Verification items for the finished model (mm, model axes). Face numbers are marked on the shaded views. A direction names the side the tool comes from. Coordinates: 2 decimals unless noted, no trailing zeros. Order: outer loops, then holes, each group sorted by start corner. A loop starts at its lowest first (then second) coordinate and runs counter-clockwise, first axis right, second up. Notation, with made-up numbers: (57.25, 57) -> (79.25, 57) arc R19 cw to (79.25, 87) -> close; hole circle Ø9 at (-7.5, -20). An arc over 180 degrees is marked (long way). Write item = value, one per line. Start each with the question number.
1. Cross-section at B-B on y = -421. Record the cut outline in (x, z), plus the area to 3 significant figures.
2. Thickness scan on line 1 along Z through (x, y) = (487, -606); line 2 along Y through (x, z) = (358, 152.5); line 3 along X through (y, z) = (-537.5, 164). Record the ranges inside material, lowest first. Write a range as from..to.
3. Cross-section at C-C on x = 64. Record the cut outline in (y, z).
4. Cross-section at A-A on z = 359.5. Record the cut outline in (x, y).
5. Go/stop test with a flat-tipped pin: P1, Ø4, axis at x = 268.5, y = -381.5, coming from the -Z side. Record where the tip stops, or that it passes through.
6. Release check for a two-part mould opening along X. For the marked faces 1, 2 and 3 record: +X half, -X half, draft (parallel to the pull), parting line (faces both ways), or undercut.
7. Set-up check for the marked faces 4 and 5: record each of +Z, -Z, +X, -X, +Y, -Y from which the full face is reachable in a straight line by a thin tool's end or side.
from build123d import *

# Parameters (mm, degrees)
SKETCH_2_W           = 559.015307906
SKETCH_2_H           = 680
EXTRUDE_2_DEPTH      = 400
SKETCH_3_OUTSIDE_W   = 754.395
SKETCH_3_OUTSIDE_H   = 875.38
SKETCH_3_OUTSIDE_W_2 = 559.015307906
SKETCH_3_OUTSIDE_H_2 = 490.432891875
CUT_EXTRUDE_1_DEPTH  = 784.744027655
SKETCH_4_W           = 559.015307906
SKETCH_4_H           = 490.432891875
EXTRUDE_3_DEPTH      = 100
SHELL_2_T            = -30
SKETCH_5_W           = 499.015307907
SKETCH_5_H           = 6
CUT_EXTRUDE_2_DEPTH  = 10
SKETCH_6_W           = 499.015307907
SKETCH_6_H           = 6
CUT_EXTRUDE_3_DEPTH  = 10
SKETCH_7_W           = 6
SKETCH_7_H           = 490.432891874
CUT_EXTRUDE_4_DEPTH  = 10


with BuildPart() as part:
    # 草图2 → 凸台-拉伸2 (new body)
    with BuildSketch(Plane(origin=(180.83794206, -79.035754343, 0), x_dir=(1, 0, 0), z_dir=(0, 0, 1))):
        with Locations((101.397699083, -216.026809528)):
            Rectangle(SKETCH_2_W, SKETCH_2_H)
    extrude(amount=EXTRUDE_2_DEPTH)

    # 草图3 outside → 切除-拉伸1 (cut, through all)
    with BuildSketch(Plane(origin=(180.83794206, -79.035754343, 400), x_dir=(1, 0, 0), z_dir=(0, 0, 1))):
        with Locations((101.3975, -216.027)):
            Rectangle(SKETCH_3_OUTSIDE_W, SKETCH_3_OUTSIDE_H)
        with Locations((101.397699083, -310.72828395)):
            Rectangle(SKETCH_3_OUTSIDE_W_2, SKETCH_3_OUTSIDE_H_2, mode=Mode.SUBTRACT)
    extrude(amount=-CUT_EXTRUDE_1_DEPTH, mode=Mode.SUBTRACT)

    # 草图4 → 凸台-拉伸3 (add)
    with BuildSketch(Plane(origin=(180.83794206, -79.035754343, 0), x_dir=(-1, 0, 0), z_dir=(0, 0, -1))):
        with Locations((-101.397699083, -310.72828395)):
            Rectangle(SKETCH_4_W, SKETCH_4_H)
    extrude(amount=EXTRUDE_3_DEPTH)

    # 抽壳2
    shell_2_openings = [part.faces().sort_by_distance(p)[0] for p in [
        (282.235641143, -389.764038294, -100),
    ]]
    offset(amount=SHELL_2_T, openings=shell_2_openings, kind=Kind.INTERSECTION)

    # 草图5 → 切除-拉伸2 (cut)
    with BuildSketch(Plane.XZ.offset(174.547592357)):
        with Locations((282.235641143, -87)):
            Rectangle(SKETCH_5_W, SKETCH_5_H)
    cut_extrude_2 = extrude(amount=-CUT_EXTRUDE_2_DEPTH, mode=Mode.SUBTRACT)

    # 草图6 → 切除-拉伸3 (cut)
    with BuildSketch(Plane.XZ.offset(174.547592357)):
        with Locations((282.235641143, -76)):
            Rectangle(SKETCH_6_W, SKETCH_6_H)
    cut_extrude_3 = extrude(amount=-CUT_EXTRUDE_3_DEPTH, mode=Mode.SUBTRACT)

    # 镜向1: 切除-拉伸2, 切除-拉伸3 across plane
    add(cut_extrude_2.mirror(Plane(origin=(0, -389.764038294, 0), x_dir=(0, 0, 1), z_dir=(0, -1, 0))), mode=Mode.SUBTRACT)
    add(cut_extrude_3.mirror(Plane(origin=(0, -389.764038294, 0), x_dir=(0, 0, 1), z_dir=(0, -1, 0))), mode=Mode.SUBTRACT)

    # 草图7 → 切除-拉伸4 (cut)
    with BuildSketch(Plane.XY.offset(400)):
        with Locations((548.743295096, -389.764038294)):
            Rectangle(SKETCH_7_W, SKETCH_7_H)
    cut_extrude_4 = extrude(amount=-CUT_EXTRUDE_4_DEPTH, mode=Mode.SUBTRACT)

    # 镜向2: 切除-拉伸4 across plane
    add(cut_extrude_4.mirror(Plane.ZY.offset(-282.235641143)), mode=Mode.SUBTRACT)


solid = part.part
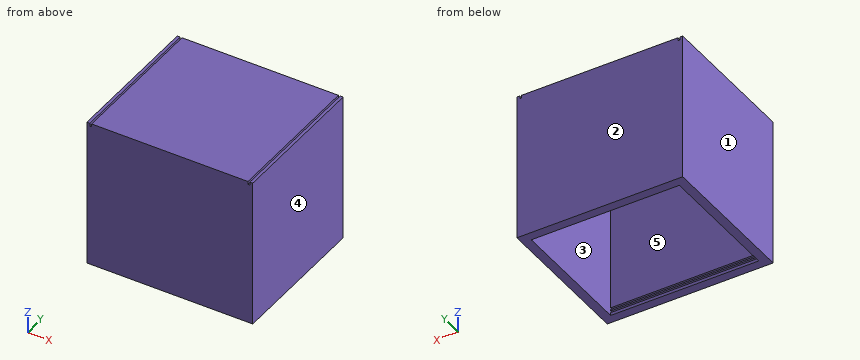
Worked out:
q1.outline = (2.73, -100) -> (32.73, -100) -> (32.73, 370) -> (531.74, 370) -> (531.74, -100) -> (561.74, -100) -> (561.74, 400) -> (551.74, 400) -> (551.74, 390) -> (545.74, 390) -> (545.74, 400) -> (18.73, 400) -> (18.73, 390) -> (12.73, 390) -> (12.73, 400) -> (2.73, 400) -> close
q1.area = 44,900 mm²
q2.line_1 = -100..-90, -84..-79, -73..400
q2.line_2 = -634.98..-604.98, -174.55..-144.55
q2.line_3 = 2.73..32.73, 531.74..561.74
q3.outline = (-634.98, -100) -> (-604.98, -100) -> (-604.98, -90) -> (-614.98, -90) -> (-614.98, -84) -> (-604.98, -84) -> (-604.98, -79) -> (-614.98, -79) -> (-614.98, -73) -> (-604.98, -73) -> (-604.98, 370) -> (-174.55, 370) -> (-174.55, -73) -> (-164.55, -73) -> (-164.55, -79) -> (-174.55, -79) -> (-174.55, -84) -> (-164.55, -84) -> (-164.55, -90) -> (-174.55, -90) -> (-174.55, -100) -> (-144.55, -100) -> (-144.55, 400) -> (-634.98, 400) -> close
q4.outline = (2.73, -634.98) -> (561.74, -634.98) -> (561.74, -144.55) -> (2.73, -144.55) -> close; hole (32.73, -604.98) -> (531.74, -604.98) -> (531.74, -174.55) -> (32.73, -174.55) -> close
q5.P1 = 370
q6.face_1 = -X half
q6.face_2 = draft
q6.face_3 = undercut
q7.face_4 = +Z, -Z, +X, +Y, -Y
q7.face_5 = -Z
